Source: CAD feature listing. Evaluate the final solid. Frame: model axes, mm. Coordinates: 2 decimals unless noted, no trailing zeros. Order: outer loops, then holes, each group sorted by start corner. A loop starts at its lowest first (then second) coordinate and runs counter-clockwise, first axis right, second up.
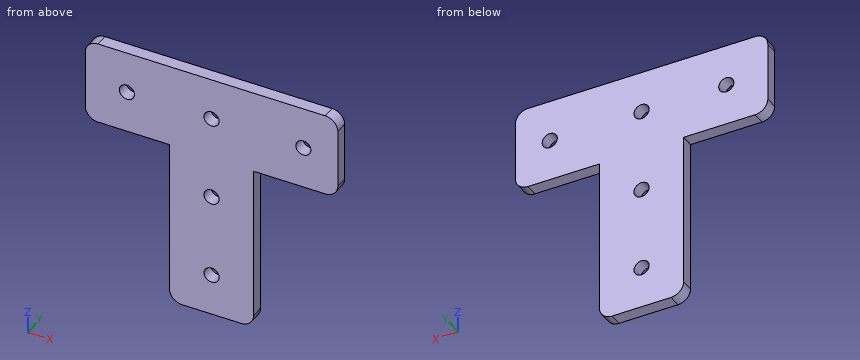
```python
from build123d import *

# Parameters (mm, degrees)
SKETCH_2_W      = 20
SKETCH_2_H      = 40
SKETCH_2_R      = 1.8
SKETCH_2_W_2    = 60
SKETCH_2_H_2    = 20
EXTRUDE_1_DEPTH = 3
FILLET_1_R      = 3


with BuildPart() as part:
    # 草图2 → 凸台-拉伸1 (new body)
    # profile 1 of 2: a face of its own
    with BuildSketch(Plane(origin=(0, 0, 0), x_dir=(1, 0, 0), z_dir=(0, 1, 0))):
        with Locations((0, 30)):
            Rectangle(SKETCH_2_W, SKETCH_2_H)
        with Locations(Location((0, 20, 0), (0, 0, 270))):
            Circle(SKETCH_2_R, mode=Mode.SUBTRACT)
        with Locations(Location((0, 40, 0), (0, 0, 270))):
            Circle(SKETCH_2_R, mode=Mode.SUBTRACT)
    # profile 2 of 2: a face of its own
    with BuildSketch(Plane(origin=(0, 0, 0), x_dir=(1, 0, 0), z_dir=(0, 1, 0))):
        Rectangle(SKETCH_2_W_2, SKETCH_2_H_2)
        with Locations(Location((0, 0, 0), (0, 0, 270))):
            Circle(SKETCH_2_R, mode=Mode.SUBTRACT)
        with Locations(Location((-20.122806929, 0, 0), (0, 0, 270))):
            Circle(SKETCH_2_R, mode=Mode.SUBTRACT)
        with Locations(Location((21.812825763, 0, 0), (0, 0, 270))):
            Circle(SKETCH_2_R, mode=Mode.SUBTRACT)
    extrude(amount=EXTRUDE_1_DEPTH)

    # 圆角1
    fillet_1_edges = [part.edges().sort_by_distance(p)[0] for p in [
        (30, 1.5, -10),
        (30, 1.5, 10),
        (-30, 1.5, 10),
        (-30, 1.5, -10),
        (-10, 1.5, -50),
        (10, 1.5, -50),
    ]]
    fillet(fillet_1_edges, radius=FILLET_1_R)


solid = part.part
```
Q1. Section query C-C on z = 0. Output: boundary loops of the cut face in (x, y), plus the area to 3 significant figures.
Solutions:
outline: (-30, 0) - (-21.92, 0) - (-21.92, 3) - (-30, 3) - close; (-18.32, 0) - (-1.8, 0) - (-1.8, 3) - (-18.32, 3) - close; (1.8, 0) - (20.01, 0) - (20.01, 3) - (1.8, 3) - close; (23.61, 0) - (30, 0) - (30, 3) - (23.61, 3) - close
area: 148 mm2
Q2. Pin query (flat end, axial travel): P1, Ø1.5, axis at y = 2, z = -28.5, coming from the -X side; P2, Ø1.5, axis at x = 14.5, y = 2, coming from the -Z side. Return the tip coordinate at first contact, or that it passes through.
Solutions:
P1: stops at x = -10
P2: stops at z = -10
Q3. Material intervals for line 1 along X through (y, z) = (2.45, 0); line 2 along X through (y, z) = (1.9, -1); line 3 along X through (y, z) = (1.35, -40), sorted ascending.
Solutions:
line 1: x = -30 to -21.92, -18.32 to -1.8, 1.8 to 20.01, 23.61 to 30
line 2: x = -30 to -21.62, -18.63 to -1.5, 1.5 to 20.32, 23.31 to 30
line 3: x = -10 to -1.8, 1.8 to 10
Q4. Section query A-A on z = -40. Output: boundary loops of the cut face in (x, y).
Solutions:
outline: (-10, 0) - (-1.8, 0) - (-1.8, 3) - (-10, 3) - close; (1.8, 0) - (10, 0) - (10, 3) - (1.8, 3) - close
Q5. Section query B-B on x = 0. Output: boundary loops of the cut face in (y, z), plus the area to 3 significant figures.
Solutions:
outline: (0, -50) - (3, -50) - (3, -41.8) - (0, -41.8) - close; (0, -38.2) - (3, -38.2) - (3, -21.8) - (0, -21.8) - close; (0, -18.2) - (3, -18.2) - (3, -1.8) - (0, -1.8) - close; (0, 1.8) - (3, 1.8) - (3, 10) - (0, 10) - close
area: 148 mm2
Q6. Section query D-D on y = 0.8. Output: boundary loops of the cut face in (x, z), plus the area to 3 significant figures.
Solutions:
outline: (-30, -7) arc R3 ccw to (-27, -10) - (-10, -10) - (-10, -47) arc R3 ccw to (-7, -50) - (7, -50) arc R3 ccw to (10, -47) - (10, -10) - (27, -10) arc R3 ccw to (30, -7) - (30, 7) arc R3 ccw to (27, 10) - (-27, 10) arc R3 ccw to (-30, 7) - close; hole circle Ø3.6 at (-20.12, 0); hole circle Ø3.6 at (0, -40); hole circle Ø3.6 at (0, -20); hole circle Ø3.6 at (0, 0); hole circle Ø3.6 at (21.81, 0)
area: 1,940 mm2
